```python
from build123d import *

# Parameters (mm, degrees)
SKETCH1_W           = 110
SKETCH1_H           = 62
BOSS_EXTRUDE1_DEPTH = 12
SKETCH2_W           = 110
SKETCH2_H           = 12
BOSS_EXTRUDE2_DEPTH = 33
BOSS_EXTRUDE3_DEPTH = 23
SKETCH7_R           = 6
CUT_EXTRUDE8_DEPTH  = 131.510535973
SKETCH9_R           = 6
CUT_EXTRUDE9_DEPTH  = 131.510535973
SKETCH10_R          = 6
CUT_EXTRUDE10_DEPTH = 129.937969582
SKETCH11_R          = 6
CUT_EXTRUDE11_DEPTH = 129.937969582
SKETCH15_W          = 60
SKETCH15_H          = 6
CUT_EXTRUDE15_DEPTH = 135.048498686
FILLET3_R           = 12
SKETCH16_R          = 15
CUT_EXTRUDE16_DEPTH = 132.030530793


with BuildPart() as part:
    # Sketch1 → Boss-Extrude1 (new body)
    with BuildSketch(Plane.XY):
        with Locations((55, 31)):
            Rectangle(SKETCH1_W, SKETCH1_H)
    extrude(amount=BOSS_EXTRUDE1_DEPTH)

    # Sketch2 → Boss-Extrude2 (add)
    with BuildSketch(Plane.XY.offset(12)):
        with Locations((55, 6)):
            Rectangle(SKETCH2_W, SKETCH2_H)
    extrude(amount=BOSS_EXTRUDE2_DEPTH)

    # Sketch3 → Boss-Extrude3 (add)
    with BuildSketch(Plane.XY.offset(12)):
        Polygon((75, 53.634363687), (35, 53.634363687), (44, 12), (66, 12), align=None)
        Polygon((80, 62), (30, 62), (30, 53.634363687), (35, 53.634363687), (75, 53.634363687), (80, 53.634363687), align=None)
    extrude(amount=BOSS_EXTRUDE3_DEPTH)

    # Sketch7 → Cut-Extrude8 (cut, through all)
    with BuildSketch(Plane.XY.offset(12)):
        with Locations((12, 50)):
            Circle(SKETCH7_R)
    extrude(amount=-CUT_EXTRUDE8_DEPTH, mode=Mode.SUBTRACT)

    # Sketch9 → Cut-Extrude9 (cut, through all)
    with BuildSketch(Plane.XY.offset(12)):
        with Locations((98, 50)):
            Circle(SKETCH9_R)
    extrude(amount=-CUT_EXTRUDE9_DEPTH, mode=Mode.SUBTRACT)

    # Sketch10 → Cut-Extrude10 (cut, through all)
    with BuildSketch(Plane(origin=(0, 12, 0), x_dir=(1, 0, 0), z_dir=(0, 1, 0))):
        with Locations(Location((12, -33, 0), (0, 0, 270))):
            Circle(SKETCH10_R)
    extrude(amount=-CUT_EXTRUDE10_DEPTH, mode=Mode.SUBTRACT)

    # Sketch11 → Cut-Extrude11 (cut, through all)
    with BuildSketch(Plane(origin=(0, 12, 0), x_dir=(1, 0, 0), z_dir=(0, 1, 0))):
        with Locations(Location((98, -33, 0), (0, 0, 270))):
            Circle(SKETCH11_R)
    extrude(amount=-CUT_EXTRUDE11_DEPTH, mode=Mode.SUBTRACT)

    # Sketch15 → Cut-Extrude15 (cut, through all)
    with BuildSketch(Plane.XY.offset(45)):
        with Locations((55, 3)):
            Rectangle(SKETCH15_W, SKETCH15_H)
    extrude(amount=-CUT_EXTRUDE15_DEPTH, mode=Mode.SUBTRACT)

    # Fillet3
    fillet3_edges = [part.edges().sort_by_distance(p)[0] for p in [
        (0, 6, 45),
        (110, 6, 45),
        (0, 62, 6),
        (110, 62, 6),
    ]]
    fillet(fillet3_edges, radius=FILLET3_R)

    # Sketch16 → Cut-Extrude16 (cut, through all)
    with BuildSketch(Plane.XY.offset(35)):
        with Locations((55, 62)):
            Circle(SKETCH16_R)
    extrude(amount=-CUT_EXTRUDE16_DEPTH, mode=Mode.SUBTRACT)


solid = part.part
```
Work out the finished part from the listing and answer in its coordinate system (mm). A direction names the side the tool comes from. Round coordinates to 2 decimals unless told otherwise and drop trailing zeros. Write each loop counter-clockwise with the first axis right and the second up, starting at its lowest first coordinate (ties: lowest second). Pieces come first, ordered by that corner, then holes.
1) A cutting plane is placed at C-C on y = 21.5. Determine the outline of the cut face in (x, z).
2) Flat-ended cylindrical pins translate along their axes: P1, Ø13, axis at x = 91, y = 29, coming from the +Z side; P2, Ø15, axis at x = 66.5, y = 45.5, coming from the +Z side; P3, Ø8, axis at x = 90.5, z = 22, coming from the +Y side; P4, Ø9.5, axis at x = 12, z = 33, coming from the -Y side. Find the tip coordinate at first contact, or state that the pin passes through.
3) A cutting plane is placed at A-A on z = 7. Determine the outline of the cut face in (x, y).
4) A cutting plane is placed at D-D on z = 14. Determine the outline of the cut face in (x, y).
5) A cutting plane is placed at B-B on x = 55. Determine the outline of the cut face in (y, z), and give its area (4 significant figures).
6) Which of the six approach directions +Z, -Z, +X, -X, +Y, -Y give full straight-line access (tool end or side, diameter ignored) to faces 4 (the face through (77, 53.634, 23)), 5 (the face through (30, 58, 23)), 6 (the face through (80, 58, 23))?
7) Determine the mould class of faces 1 (the face through (25, 3, 23)), 2 (the face through (0, 19, 9)), 3 (the face through (70.437, 32.526, 23.339)) for opening direction X: pulls with the +X half, pulls with the -X half, needs draft (parallel to the pull), parting line crosses it, or undercut.
8) Consider probe 1 along X at (y, z) = (3, 33); probe 2 along Y at (x, z) = (12, 8.25); probe 3 along X at (y, z) = (9, 33). Determine where each line is inside the solid, lowest interval first.
Entries:
1. outline: (0, 0) - (110, 0) - (110, 12) - (68.05, 12) - (68.05, 35) - (41.95, 35) - (41.95, 12) - (0, 12) - close
2. P1: stops at z = 12
2. P2: stops at z = 35
2. P3: stops at y = 12
2. P4: passes through
3. outline: (0, 0) - (25, 0) - (25, 6) - (85, 6) - (85, 0) - (110, 0) - (110, 50) arc R12 ccw to (98, 62) - (70, 62) arc R15 cw to (40, 62) - (12, 62) arc R12 ccw to (0, 50) - close; hole circle Ø12 at (12, 50); hole circle Ø12 at (98, 50)
4. outline: (0, 0) - (25, 0) - (25, 6) - (85, 6) - (85, 0) - (110, 0) - (110, 12) - (66, 12) - (75, 53.63) - (80, 53.63) - (80, 62) - (70, 62) arc R15 cw to (40, 62) - (30, 62) - (30, 53.63) - (35, 53.63) - (44, 12) - (0, 12) - close
5. outline: (6, 0) - (47, 0) - (47, 35) - (12, 35) - (12, 45) - (6, 45) - close
5. area: 1,495 mm2
6. face 4: +Z, +X
6. face 5: +Z, -X, +Y
6. face 6: +Z, +X, +Y
7. face 1: undercut
7. face 2: pulls with the -X half
7. face 3: pulls with the +X half
8. probe 1: x = 0 to 6, 18 to 25, 85 to 92, 104 to 110
8. probe 2: y = 0 to 44, 56 to 62
8. probe 3: x = 0 to 6, 18 to 92, 104 to 110
